from build123d import *

# Parameters (mm, degrees)
SKETCH1_W           = 127
SKETCH1_H           = 88.9
BOSS_EXTRUDE1_DEPTH = 31.75
SHELL1_T            = -2.54
SKETCH3_R           = 3.175
CUT_EXTRUDE2_DEPTH  = 31.75
SKETCH4_W           = 38.1
SKETCH4_H           = 26.035
CUT_EXTRUDE3_DEPTH  = 31.75
SKETCH5_W           = 25.4
SKETCH5_H           = 26.035
CUT_EXTRUDE4_DEPTH  = 31.75


with BuildPart() as part:
    # Sketch1 → Boss-Extrude1 (new body)
    with BuildSketch(Plane(origin=(0, 0, 0), x_dir=(1, 0, 0), z_dir=(0, 1, 0))):
        with Locations((63.5, 44.45)):
            Rectangle(SKETCH1_W, SKETCH1_H)
    extrude(amount=BOSS_EXTRUDE1_DEPTH)

    # Shell1
    shell1_openings = [part.faces().sort_by_distance(p)[0] for p in [
        (63.5, 31.75, -44.45),
    ]]
    offset(amount=SHELL1_T, openings=shell1_openings, kind=Kind.INTERSECTION)

    # Sketch3 → Cut-Extrude2 (cut)
    with BuildSketch(Plane(origin=(127, 0, 0), x_dir=(0, 0, -1), z_dir=(1, 0, 0))):
        with Locations((12.7, 25.4)):
            Circle(SKETCH3_R)
        with Locations((76.2, 25.4)):
            Circle(SKETCH3_R)
    cut_extrude2 = extrude(amount=-CUT_EXTRUDE2_DEPTH, mode=Mode.SUBTRACT)

    # Mirror2: Cut-Extrude2 across plane
    add(cut_extrude2.mirror(Plane(origin=(63.5, 0, 0), x_dir=(0, 0, 1), z_dir=(1, 0, 0))), mode=Mode.SUBTRACT)

    # Sketch4 → Cut-Extrude3 (cut)
    with BuildSketch(Plane.XY):
        with Locations((99.06, 18.7325)):
            Rectangle(SKETCH4_W, SKETCH4_H)
    extrude(amount=-CUT_EXTRUDE3_DEPTH, mode=Mode.SUBTRACT)

    # Sketch5 → Cut-Extrude4 (cut)
    with BuildSketch(Plane(origin=(0, 0, -88.9), x_dir=(-1, 0, 0), z_dir=(0, 0, -1))):
        with Locations((-53.34, 18.7325)):
            Rectangle(SKETCH5_W, SKETCH5_H)
    extrude(amount=-CUT_EXTRUDE4_DEPTH, mode=Mode.SUBTRACT)


solid = part.part
For this review, take the finished solid that the model builds, in its own axes (mm). A direction names the side the tool comes from. Round coordinates to 2 decimals unless told otherwise and drop trailing zeros. Write each loop counter-clockwise with the first axis right and the second up, starting at its lowest first coordinate (ties: lowest second). Pieces come first, ordered by that corner, then holes. Notation, with made-up numbers: M -25.5,18 L -5.5,18 A30 cw -5.5,43 Z; hole C 50.25,64.5 d2. An arc over 180 degrees is marked long. Write item = value, one per line. Start each with the question number.
(1) We need section D-D (z = -52). Give the boundary of the cut face in (x, y).
(2) The part is to be moulded in two halves that separate along Z. For faces 6 (the face through (1.25, 28.55, -75.79)), 7 (the face through (126, 31.75, -61)), 8 (the face through (2.54, 17, -44)), 9 (the face through (48, 16, 0)), say which applies: +Z half, -Z half, draft (parallel to the pull), parting line (faces both ways), or undercut.
(3) We need section B-B (z = -76.2). Give the boundary of the cut face in (x, y) (3 decimals), then the cut area to 3 significant figures.
(4) We need section C-C (y = 25.4). Give the number of separate pieces and of enclosed holes in the cut face, then the cut area to 3 significant figures.
(5) We need section A-A (y = 10.5). Give the boundary of the cut face in (x, z).
(6) For faces 1 (the face through (63, 2.54, -45)), 2 (the face through (125.75, 28.55, -75.79)), 3 (the face through (40.64, 19, -88)), 4 (the face through (1, 31.75, -35)), 5 (the face through (99, 5.715, -1)), list the 3-axis set-ups (+Z, -Z, +X, -X, +Y, -Y) from which the entire face can be reached by the end or side of a thin tool; tool diameter is ignored.
(7) Clearance check with flat-ended pins moving along their axes: pin 1 Ø9 at (x, y) = (39, 17) entering from +Z; pin 2 Ø1.3 at (x, z) = (107.5, -1.5) entering from +Y (3 decimals); pin 3 Ø1 at (x, z) = (112.5, -9.5) entering from +Y. State where each tip first meets the part, or that it passes through.
(8) For line 1 along Z through (x, y) = (125, 25); line 2 along Z through (x, y) = (0.95, 25.4) (3 decimals); line 3 along X through (y, z) = (13, -52), list the stretches that pass through material, from the lowest coordinate up.
Results found:
q1.outline = M 0,0 L 127,0 L 127,31.75 L 124.46,31.75 L 124.46,2.54 L 2.54,2.54 L 2.54,31.75 L 0,31.75 Z
q2.face_6 = undercut
q2.face_7 = draft
q2.face_8 = undercut
q2.face_9 = +Z half
q3.outline = M 0,0 L 127,0 L 127,22.225 L 124.46,22.225 L 124.46,2.54 L 2.54,2.54 L 2.54,22.225 L 0,22.225 Z; M 0,28.575 L 2.54,28.575 L 2.54,31.75 L 0,31.75 Z; M 124.46,28.575 L 127,28.575 L 127,31.75 L 124.46,31.75 Z
q3.area = 439 mm²
q4.separate_pieces = 6
q4.enclosed_holes = 0
q4.area = 845 mm²
q5.outline = M 0,-88.9 L 40.64,-88.9 L 40.64,-86.36 L 2.54,-86.36 L 2.54,-2.54 L 80.01,-2.54 L 80.01,0 L 0,0 Z; M 66.04,-88.9 L 127,-88.9 L 127,0 L 118.11,0 L 118.11,-2.54 L 124.46,-2.54 L 124.46,-86.36 L 66.04,-86.36 Z
q6.face_1 = +Y
q6.face_2 = +X, -X
q6.face_3 = -Z, +Y
q6.face_4 = +Z, -Z, +X, -X, +Y
q6.face_5 = +Z, +Y
q7.pin_1 = 0
q7.pin_2 = 5.715
q7.pin_3 = 2.54
q8.line_1 = -88.9 to -79.35, -73.05 to -15.85, -9.55 to 0
q8.line_2 = -88.9 to -79.375, -73.025 to -15.875, -9.525 to 0
q8.line_3 = 0 to 2.54, 124.46 to 127
